CAD build for the part. Positions are in the model's coordinates, mm. Face numbers are marked on the shaded views. A direction names the side the tool comes from. Coordinates: 2 decimals unless noted, no trailing zeros. Write each loop counter-clockwise with the first axis right and the second up, starting at its lowest first coordinate (ties: lowest second). Pieces come first, ordered by that corner, then holes. Notation, with made-up numbers: M 17.5,41 L 76.5,41 A22 ccw 76.5,67 Z; hole C 79,67.25 d5. An arc over 180 degrees is marked long. Answer as CSV lines item,"result". Start each with the question number.
```python
from build123d import *

# Parameters (mm, degrees)
SKETCH1_W           = 69.85
SKETCH1_H           = 31.75
BOSS_EXTRUDE1_DEPTH = 2.54
SKETCH2_W           = 3.81
SKETCH2_H           = 29.21
BOSS_EXTRUDE2_DEPTH = 9.652
SKETCH3_R           = 5.08
CUT_EXTRUDE1_DEPTH  = 10.16
CUT_EXTRUDE2_DEPTH  = 10.16
FILLET1_R           = 2.54
FILLET2_R           = 2.54
SKETCH11_R          = 3.81
CUT_EXTRUDE3_DEPTH  = 10.16


with BuildPart() as part:
    # Sketch1 → Boss-Extrude1 (new body)
    with BuildSketch(Plane.XY):
        Rectangle(SKETCH1_W, SKETCH1_H)
    extrude(amount=BOSS_EXTRUDE1_DEPTH)

    # Sketch2 → Boss-Extrude2 (add)
    with BuildSketch(Plane(origin=(0, 0, 0), x_dir=(-1, 0, 0), z_dir=(0, 0, -1))):
        with Locations((27.700292401, 0)):
            Rectangle(SKETCH2_W, SKETCH2_H)
    extrude(amount=BOSS_EXTRUDE2_DEPTH)

    # Sketch3 → Cut-Extrude1 (cut)
    with BuildSketch(Plane(origin=(-25.795292401, 0, 0), x_dir=(0, 0, -1), z_dir=(1, 0, 0))):
        with Locations((9.652, 0)):
            Circle(SKETCH3_R)
    extrude(amount=-CUT_EXTRUDE1_DEPTH, mode=Mode.SUBTRACT)

    # Sketch9 → Cut-Extrude2 (cut)
    with BuildSketch(Plane.XY.offset(2.54)):
        with BuildLine():
            Line((0, 15.875), (34.925, 15.875))
            Line((34.925, 15.875), (34.925, 8.255))
            ThreePointArc((34.925, 8.255), (17.731940388, 13.29993511), (0, 15.875))
        make_face()
        with BuildLine():
            Line((0, -15.875), (34.925, -15.875))
            Line((34.925, -15.875), (34.925, -8.255))
            ThreePointArc((34.925, -8.255), (17.731940388, -13.29993511), (0, -15.875))
        make_face()
    extrude(amount=-CUT_EXTRUDE2_DEPTH, mode=Mode.SUBTRACT)

    # Fillet1
    fillet1_edges = [part.edges().sort_by_distance(p)[0] for p in [
        (-34.925, 15.875, 1.27),
        (-34.925, -15.875, 1.27),
    ]]
    fillet(fillet1_edges, radius=FILLET1_R)

    # Fillet2
    fillet2_edges = [part.edges().sort_by_distance(p)[0] for p in [
        (34.925, 8.255, 1.27),
        (34.925, -8.255, 1.27),
    ]]
    fillet(fillet2_edges, radius=FILLET2_R)

    # Sketch11 → Cut-Extrude3 (cut)
    with BuildSketch(Plane.XY.offset(2.54)):
        with Locations((24.765, 0)):
            Circle(SKETCH11_R)
    extrude(amount=-CUT_EXTRUDE3_DEPTH, mode=Mode.SUBTRACT)


solid = part.part
```
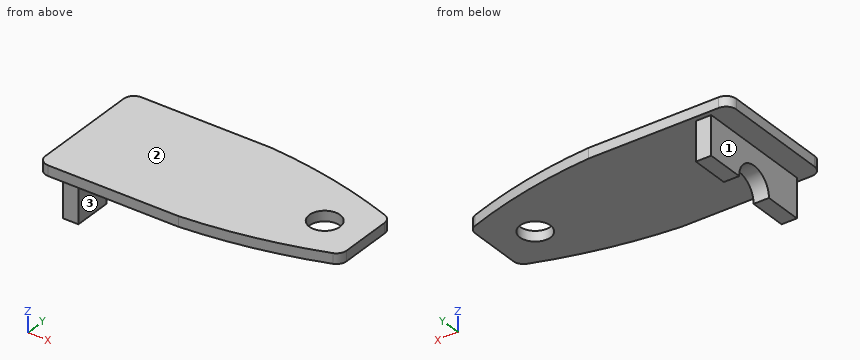
1) Band-saw the part on C-C, the plane z = -7. List the corners of the cut face in (x, y) (3 decimals), plus the area to 3 significant figures.
2) Band-saw the part on A-A, the plane y = 0. List the corners of the cut face in (x, z) (3 decimals), plus the area to 3 significant figures.
3) Band-saw the part on D-D, the plane y = 12. List the corners of the cut face in (x, z) (3 decimals), plus the area to 3 significant figures.
4) Probe L1, parallel to X at y = 0.5, z = -2; L2, parallel to Z at x = -7, y = -0.5; L3, parallel to Y at x = -28, z = -6.25 (3 decimals). List the from-to ranges inside material, lowest first. Write a range as [from, to].
5) Tool access for the marked faces 1, 2 and 3: list every direction of +Z, -Z, +X, -X, +Y, -Y with a clear straight run to the whole face (end or side of a thin tool).
6) Band-saw the part on B-B, the plane z = 0.75. List the corners of the cut face in (x, y) (3 decimals), plus the area to 3 significant figures.
7) Pin check, flat tips, straight feed: P1, Ø2, axis at x = -13.5, z = -0.5, coming from the -Y side (3 decimals); P2, Ø4.5, axis at x = 24.765, y = 0, coming from the +Z side; P3, Ø5, axis at y = 0, z = -4.5, coming from the -X side; P4, Ø1.9, axis at x = -28.5, z = -7, coming from the -Y side (3 decimals). Stop position of each tip, or through.
Result sheet:
1,outline,"M -29.605,-14.605 L -25.795,-14.605 L -25.795,-4.333 L -29.605,-4.333 Z; M -29.605,4.333 L -25.795,4.333 L -25.795,14.605 L -29.605,14.605 Z"
1,area,"78.3 mm²"
2,outline,"M -34.925,0 L -29.605,0 L -29.605,-4.572 L -25.795,-4.572 L -25.795,0 L 20.955,0 L 20.955,2.54 L -34.925,2.54 Z; M 28.575,0 L 34.925,0 L 34.925,2.54 L 28.575,2.54 Z"
2,area,"175 mm²"
3,outline,"M -34.925,0 L -29.605,0 L -29.605,-9.652 L -25.795,-9.652 L -25.795,0 L 23.122,0 L 23.122,2.54 L -34.925,2.54 Z"
3,area,"184 mm²"
4,L1,"x = [-29.61, -25.8]"
4,L2,"z = [0, 2.54]"
4,L3,"y = [-14.605, -3.773], [3.773, 14.605]"
5,face 1,"-Z, -X, +Y, -Y"
5,face 2,"+Z, +X, -X, +Y, -Y"
5,face 3,"-Z, +X, +Y, -Y"
6,outline,"M -34.925,-13.335 A2.54 ccw -32.385,-15.875 L 0,-15.875 A127 ccw 33.237,-8.869 A2.54 ccw 34.925,-6.476 L 34.925,6.476 A2.54 ccw 33.237,8.869 A127 ccw 0,15.875 L -32.385,15.875 A2.54 ccw -34.925,13.335 Z; hole C 24.765,0 d7.62"
6,area,"1,960 mm²"
7,P1,"stops at y = -15.875"
7,P2,"passes through"
7,P3,"stops at x = -29.61"
7,P4,"stops at y = -14.605"
